```python
from build123d import *

# Parameters (mm, degrees)
F0_W     = 519.4771289825
F0_H     = 145.3515
F0_W_2   = 78.8426995277
F0_W_3   = 543.9197421074
F0_W_4   = 64.8887902498
F0_W_5   = 117.8393810987
F0_H_2   = 64.897
F0_H_3   = 145.9111776203
F0_W_6   = 64.897
F0_H_4   = 132.8892552004
F0_H_5   = 154.8609585657
F0_W_7   = 83.3352580338
F1_DEPTH = 76.2
F2_R     = 190.5
F3_DEPTH = 76.2
F4_R     = 190.5
F5_DEPTH = 76.2
F6_W     = 560.091412735
F6_H     = 355.6
F7_DEPTH = 50.8
F8_W     = 115.9408456802
F8_H     = 355.6
F9_DEPTH = 355.6


with BuildPart() as f1:
    # F0 (on Top) → F1 (new body)
    with BuildSketch(Plane.XY):
        with Locations((372.2674846649, 44.8714789324)):
            Rectangle(F0_W, F0_H)
        Polygon((112.5289201736, -160.693526268), (112.5289201736, -27.8042710676), (112.5289201736, 117.5472289324), (47.6401299238, 117.5472289324), (47.6401299238, -28.3639486879), (47.6401299238, -160.693526268), align=None)
        with Locations((671.4273989201, 44.8714789324)):
            Rectangle(F0_W_2, F0_H)
        with Locations((982.8086197376, 44.8714789324)):
            Rectangle(F0_W_3, F0_H)
        with Locations((80.0845250487, 255.1199789324)):
            Rectangle(F0_W_4, F0_H)
        Polygon((112.5289201736, 327.7957289324), (112.5289201736, 182.4442289324), (632.0060491562, 182.4442289324), (632.0060491562, 327.7957289324), (539.4007488251, 327.7957289324), align=None)
        with Locations((-11.2795606256, 149.9957289324)):
            Rectangle(F0_W_5, F0_H_2)
        with Locations((-11.2795606256, 44.5916401222)):
            Rectangle(F0_W_5, F0_H_3)
        with Locations((1287.2169907913, 44.8714789324)):
            Rectangle(F0_W_6, F0_H)
        with Locations((1287.2169907913, -94.2488986678)):
            Rectangle(F0_W_6, F0_H_4)
        Polygon((632.0060491562, 327.7957289324), (632.0060491562, 182.4442289324), (710.8487486839, 182.4442289324), (710.8487486839, 327.7957289324), (666.4007488251, 327.7957289324), align=None)
        with Locations((80.0845250487, 405.2262082152)):
            Rectangle(F0_W_4, F0_H_5)
        with Locations((-11.2795606256, 255.1199789324)):
            Rectangle(F0_W_5, F0_H)
        with Locations((1361.3331198082, 44.8714789324)):
            Rectangle(F0_W_7, F0_H)
        with Locations((982.8086197376, 255.1199789324)):
            Rectangle(F0_W_3, F0_H)
        with Locations((1361.3331198082, 149.9957289324)):
            Rectangle(F0_W_7, F0_H_2)
        with Locations((1287.2169907913, 255.1199789324)):
            Rectangle(F0_W_6, F0_H)
        with Locations((1361.3331198082, 255.1199789324)):
            Rectangle(F0_W_7, F0_H)
        with Locations((1287.2169907913, 405.2262082152)):
            Rectangle(F0_W_6, F0_H_5)
    extrude(amount=F1_DEPTH)

    # F2 (on face) → F3 (join)
    with BuildSketch(Plane(origin=(0, 482.6566874981, 0), x_dir=(-1, 0, 0), z_dir=(0, 1, 0))):
        with Locations((-80.1467373967, 39.5456925035)):
            Circle(F2_R)
        with Locations((-1288.2950305939, 39.5456925035)):
            Circle(F2_R)
    extrude(amount=F3_DEPTH)

    # F4 (on face) → F5 (join)
    with BuildSketch(Plane.XZ.offset(160.693526268)):
        with Locations((1283.8026285172, 38.1)):
            Circle(F4_R)
        with Locations((87.3321071267, 38.1)):
            Circle(F4_R)
    extrude(amount=F5_DEPTH)

    # F6 (on face) → F7 (join)
    with BuildSketch(Plane(origin=(0, 0, 0), x_dir=(1, 0, 0), z_dir=(0, 0, -1))):
        with Locations((1122.9550424576, -149.9957289324)):
            Rectangle(F6_W, F6_H)
    extrude(amount=F7_DEPTH)

    # F8 (on face) → F9 (join)
    with BuildSketch(Plane(origin=(0, 0, -50.8), x_dir=(1, 0, 0), z_dir=(0, 0, -1))):
        with Locations((1345.030325985, -149.9957289324)):
            Rectangle(F8_W, F8_H)
    extrude(amount=F9_DEPTH)


solid = f1.part
```
Design review of the part built by this model. Coordinates are the model's own, in mm. A direction names the side the tool comes from. Coordinates: 2 decimals unless noted, no trailing zeros. Loops run counter-clockwise (first coordinate to the right, second up) from the corner with the lowest first, then second, coordinate; pieces in that order, holes last. Notation, with made-up numbers: (7, 34.25) - (27, 34.25) arc R15 ccw to (27, 41.25) - close; hole circle Ø3 at (-13.5, 61.5). An arc over 180 degrees is marked (long way). Use CSV: the item, a comma, the result in double quotes. Start each with the question number.
1) Consider section B-B on z = -88.5. Write out the cut boundary in (x, y), then the cut area to 3 significant figures.
2) Consider section D-D on x = 197. Write out the cut boundary in (y, z), then the cut area to 3 significant figures.
3) Wall thickness on L1, parallel to Y at x = 19, z = 34.5; L2, parallel to Y at x = 1392, z = -2; L3, parallel to X at y = 368, z = 11: over which ranges is each line inside the solid? List them lowest first. Write a range as from..to.
4) Tool access review of faces 4 (the flat face through (1403.001, 152, -162)), 5 (the flat face through (675, 182.444, 38)), 6 (the flat face through (112.529, 404, 38)), 7 (the flat face through (1062, 148, -50.8)): name each direction out of +Z, -Z, +X, -X, +Y, -Y from which nothing blocks a thin tool from reaching the whole face with its end or side.
5) For pin 1 Ø8 at (x, y) = (494.5, 110.5) entering from +Z; pin 2 Ø23 at (y, z) = (140.5, 32.5) entering from -X; pin 3 Ø23 at (y, z) = (437, 39) entering from +X, all flat-tipped, find the tip position at first contact; note any pin that passes through.
6) Consider section C-C on y = 442.5. Write out the cut boundary in (x, z).
7) The part is to be moulded in two halves that separate along X. For faces 1 (the flat face through (47.64, 406, 38)), 2 (the flat face through (380, 94, 0)), 3 (the flat face through (946, -27.804, -39)), say which applies: +X half, -X half, draft (parallel to the pull), parting line (faces both ways), or undercut.
8) Consider section A-A on x = 409. Write out the cut boundary in (y, z), then the cut area to 3 significant figures.
Geometry says:
1,outline,"(-60.9, 482.66) - (221.19, 482.66) - (221.19, 558.86) - (-60.9, 558.86) - close; (-55.01, -236.89) - (229.68, -236.89) - (229.68, -160.69) - (-55.01, -160.69) - close; (1141.46, -236.89) - (1426.15, -236.89) - (1426.15, -160.69) - (1141.46, -160.69) - close; (1147.25, 482.66) - (1429.34, 482.66) - (1429.34, 558.86) - (1147.25, 558.86) - close; (1287.06, -27.8) - (1403, -27.8) - (1403, 327.8) - (1287.06, 327.8) - close"
1,area,"128,000 mm^2"
2,outline,"(-236.89, -117.67) - (-160.69, -117.67) - (-160.69, 193.87) - (-236.89, 193.87) - close; (-27.8, 0) - (117.55, 0) - (117.55, 76.2) - (-27.8, 76.2) - close; (182.44, 0) - (327.8, 0) - (327.8, 76.2) - (182.44, 76.2) - close; (482.66, -110.91) - (558.86, -110.91) - (558.86, 190) - (482.66, 190) - close"
2,area,"68,800 mm^2"
3,L1,"-236.89..-160.69, -28.36..327.8, 482.66..558.86"
3,L2,"-236.89..-160.69, -27.8..327.8, 482.66..558.86"
3,L3,"47.64..112.53, 1254.77..1319.67"
4,face 4,"+Z, -Z, +X"
4,face 5,"+Z"
4,face 6,"+Z, -Z"
4,face 7,"-Z, -X"
5,pin 1,"z = 76.2"
5,pin 2,"x = -70.2"
5,pin 3,"x = 1319.67"
6,outline,"(47.64, 0) - (112.53, 0) - (112.53, 76.2) - (47.64, 76.2) - close; (1254.77, 0) - (1319.67, 0) - (1319.67, 76.2) - (1254.77, 76.2) - close"
7,face 1,"-X half"
7,face 2,"draft"
7,face 3,"undercut"
8,outline,"(-27.8, 0) - (117.55, 0) - (117.55, 76.2) - (-27.8, 76.2) - close; (182.44, 0) - (327.8, 0) - (327.8, 76.2) - (182.44, 76.2) - close"
8,area,"22,200 mm^2"
